Build history of the part. All positions in model axes, mm. Face numbers are marked on the shaded views. Give positions to 0.01 mm unless a question says otherwise; leave off trailing zeros. Loops run counter-clockwise (first coordinate to the right, second up) from the corner with the lowest first, then second, coordinate; pieces in that order, holes last. Notation, with made-up numbers: M 79,67.5 L 86,67.5 A8 cw 86,80.5 Z; hole C 80,-39 d3. An arc over 180 degrees is marked long. Answer as a JSON object with one key per item and string values. Group by question number.
1. Slice it at B-B (z = 11). List the corners of the cut face in (x, y).
2. Slice it at D-D (x = 37.5). List the corners of the cut face in (y, z), then the cut area to 3 significant figures.
3. Slice it at C-C (y = 0). List the corners of the cut face in (x, z).
4. Slice it at A-A (x = -22.5). List the corners of the cut face in (y, z), then the cut area to 3 significant figures.
5. Mould opens along Y. For the marked faces 1, 2 and 3 say: released by +Y, released by -Y, zero draft, split by the parting line, or undercut.
6. Drop flat-ended pins along their axis: pin 1 Ø5 at (x, z) = (-19, 8.5) entering from +Y; pin 2 Ø4 at (y, z) = (-22.5, 22) entering from -X; pin 3 Ø5 at (y, z) = (-45, 26) entering from -X; pin 4 Ø1 at (x, y) = (-4.5, -82) entering from -Z. Give the stop position or say it passes through.
7. Drill centre lines: line 1 along Y through (x, z) = (22.5, 23.75); line 2 along Y through (x, z) = (-33, 26); line 3 along Y through (x, z) = (17.5, 27.5). Where is each one in solid material? Low to high. Write a range as [from, to].
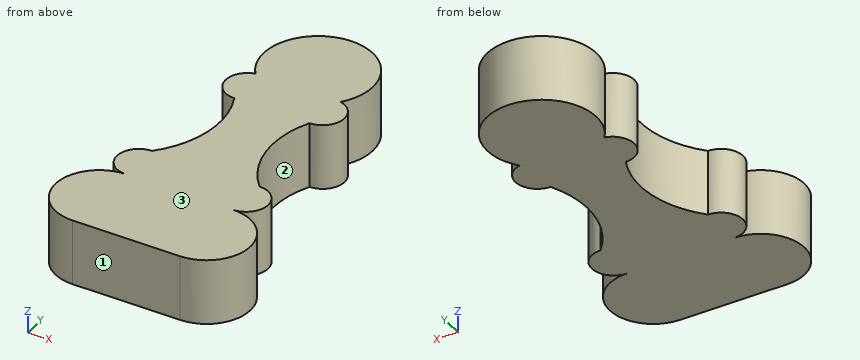
from build123d import *

# Parameters (mm, degrees)
BOSS_EXTRUDE3_DEPTH = 30


with BuildPart() as part:
    # Sketch1 → Boss-Extrude3 (new body)
    with BuildSketch(Plane.XY):
        with BuildLine():
            ThreePointArc((19.796695306, -15.267313286), (0, 25), (-19.796695306, -15.267313286))
            ThreePointArc((-19.796695306, -15.267313286), (-27.432946872, -26.156099663), (-17.5, -35))
            ThreePointArc((-17.5, -35), (-13.564166187, -61.152875072), (-25, -85))
            ThreePointArc((-25, -85), (-35, -95), (-25, -105))
            ThreePointArc((-25, -105), (-45, -125), (-25, -145))
            Line((-25, -145), (25, -145))
            ThreePointArc((25, -145), (45, -125), (25, -105))
            ThreePointArc((25, -105), (35, -95), (25, -85))
            ThreePointArc((25, -85), (13.564166187, -61.152875072), (17.5, -35))
            ThreePointArc((17.5, -35), (27.432946872, -26.156099663), (19.796695306, -15.267313286))
        make_face()
    extrude(amount=BOSS_EXTRUDE3_DEPTH)


solid = part.part
Established:
{
 "1": {"outline": "M -25,-145 L 25,-145 A20 ccw 25,-105 A10 ccw 25,-85 A45 cw 17.5,-35 A10 ccw 19.8,-15.27 A25 ccw long -19.8,-15.27 A10 ccw -17.5,-35 A45 cw -25,-85 A10 ccw -25,-105 A20 ccw Z"},
 "2": {"outline": "M -140.61,0 L -109.39,0 L -109.39,30 L -140.61,30 Z", "area": "937 mm^2"},
 "3": {"outline": "M -25,0 L 25,0 L 25,30 L -25,30 Z"},
 "4": {"outline": "M -145,0 L -82.05,0 L -82.05,30 L -145,30 Z; M -33.66,0 L -16.34,0 L -16.34,30 L -33.66,30 Z; M -10.9,0 L 10.9,0 L 10.9,30 L -10.9,30 Z", "area": "3,060 mm^2"},
 "5": {"face 1": "released by -Y", "face 2": "undercut", "face 3": "zero draft"},
 "6": {"pin 1": "stops at y = 18.78", "pin 2": "stops at x = -27.49", "pin 3": "stops at x = -14.69", "pin 4": "stops at z = 0"},
 "7": {"line 1": "y = [-145, -82.05], [-33.66, -16.34], [-10.9, 10.9]", "line 2": "y = [-143.33, -106.67], [-101, -89]", "line 3": "y = [-145, -73.96], [-35, 17.85]"}
}
